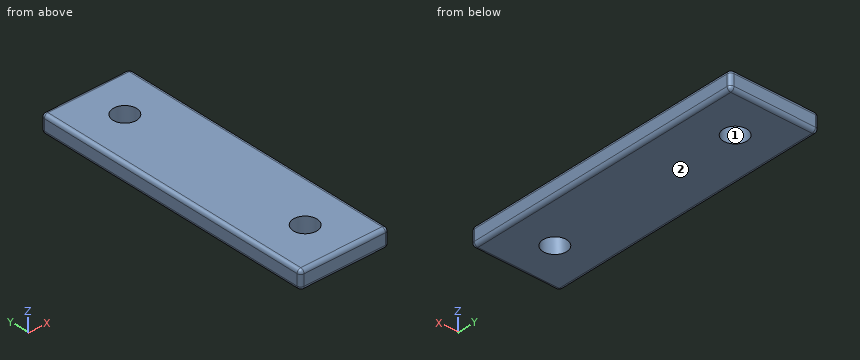
from build123d import *

# Parameters (mm, degrees)
SKETCH1_W           = 48
SKETCH1_H           = 155
BOSS_EXTRUDE1_DEPTH = 10
FILLET1_R           = 2
FILLET2_R           = 2
SKETCH2_R           = 6.4
CUT_EXTRUDE1_DEPTH  = 82.74503043


with BuildPart() as part:
    # Sketch1 → Boss-Extrude1 (new body)
    with BuildSketch(Plane.XY):
        Rectangle(SKETCH1_W, SKETCH1_H)
    extrude(amount=BOSS_EXTRUDE1_DEPTH)

    # Fillet1
    fillet1_edges = [part.edges().sort_by_distance(p)[0] for p in [
        (-24, 0, 10),
        (0, -77.5, 10),
        (24, 0, 10),
        (0, -77.5, 0),
        (-24, 0, 0),
        (0, 77.5, 0),
        (24, 0, 0),
        (0, 77.5, 10),
    ]]
    fillet(fillet1_edges, radius=FILLET1_R)

    # Fillet2
    # the kernel refuses this fillet: 2 mm, written as the material it takes off along each edge
    with BuildSketch(Plane(origin=(-22, 75.5, 8), x_dir=(0, 1, 0), z_dir=(-1, 0, 0))) as fillet2_piece_1_section:
        Polygon((0, 0), (FILLET2_R, 0), (FILLET2_R, -FILLET2_R), (0, -FILLET2_R), align=None)
    fillet2_piece_1 = extrude(amount=FILLET2_R, mode=Mode.PRIVATE)
    fillet2_piece_1 = fillet2_piece_1 - Plane(origin=(-22, 75.5, 8), x_dir=(0, -0.7071067811865475, -0.7071067811865475), z_dir=(-1, 0, 0)) * Sphere(FILLET2_R, mode=Mode.PRIVATE)
    add(fillet2_piece_1, mode=Mode.SUBTRACT)
    with BuildSketch(Plane(origin=(22, 75.5, 8), x_dir=(0, 1, 0), z_dir=(1, 0, 0))) as fillet2_piece_2_section:
        Polygon((0, 0), (FILLET2_R, 0), (FILLET2_R, FILLET2_R), (0, FILLET2_R), align=None)
    fillet2_piece_2 = extrude(amount=FILLET2_R, mode=Mode.PRIVATE)
    fillet2_piece_2 = fillet2_piece_2 - Plane(origin=(22, 75.5, 8), x_dir=(0, -0.7071067811865475, -0.7071067811865475), z_dir=(1, 0, 0)) * Sphere(FILLET2_R, mode=Mode.PRIVATE)
    add(fillet2_piece_2, mode=Mode.SUBTRACT)
    with BuildSketch(Plane(origin=(-22, -75.5, 8), x_dir=(-1, 0, 0), z_dir=(0, -1, 0))) as fillet2_piece_3_section:
        Polygon((0, 0), (FILLET2_R, 0), (FILLET2_R, -FILLET2_R), (0, -FILLET2_R), align=None)
    fillet2_piece_3 = extrude(amount=FILLET2_R, mode=Mode.PRIVATE)
    fillet2_piece_3 = fillet2_piece_3 - Plane(origin=(-22, -75.5, 8), x_dir=(0.7071067811865475, 0, -0.7071067811865475), z_dir=(0, -1, 0)) * Sphere(FILLET2_R, mode=Mode.PRIVATE)
    add(fillet2_piece_3, mode=Mode.SUBTRACT)
    with BuildSketch(Plane(origin=(22, -75.5, 8), x_dir=(1, 0, 0), z_dir=(0, -1, 0))) as fillet2_piece_4_section:
        Polygon((0, 0), (FILLET2_R, 0), (FILLET2_R, FILLET2_R), (0, FILLET2_R), align=None)
    fillet2_piece_4 = extrude(amount=FILLET2_R, mode=Mode.PRIVATE)
    fillet2_piece_4 = fillet2_piece_4 - Plane(origin=(22, -75.5, 8), x_dir=(-0.7071067811865475, 0, -0.7071067811865475), z_dir=(0, -1, 0)) * Sphere(FILLET2_R, mode=Mode.PRIVATE)
    add(fillet2_piece_4, mode=Mode.SUBTRACT)
    with BuildSketch(Plane(origin=(22, -75.5, 2), x_dir=(1, 0, 0), z_dir=(0, -1, 0))) as fillet2_piece_5_section:
        Polygon((0, 0), (FILLET2_R, 0), (FILLET2_R, -FILLET2_R), (0, -FILLET2_R), align=None)
    fillet2_piece_5 = extrude(amount=FILLET2_R, mode=Mode.PRIVATE)
    fillet2_piece_5 = fillet2_piece_5 - Plane(origin=(22, -75.5, 2), x_dir=(-0.7071067811865475, 0, 0.7071067811865475), z_dir=(0, -1, 0)) * Sphere(FILLET2_R, mode=Mode.PRIVATE)
    add(fillet2_piece_5, mode=Mode.SUBTRACT)
    with BuildSketch(Plane(origin=(-22, -75.5, 2), x_dir=(-1, 0, 0), z_dir=(0, -1, 0))) as fillet2_piece_6_section:
        Polygon((0, 0), (FILLET2_R, 0), (FILLET2_R, FILLET2_R), (0, FILLET2_R), align=None)
    fillet2_piece_6 = extrude(amount=FILLET2_R, mode=Mode.PRIVATE)
    fillet2_piece_6 = fillet2_piece_6 - Plane(origin=(-22, -75.5, 2), x_dir=(0.7071067811865475, 0, 0.7071067811865475), z_dir=(0, -1, 0)) * Sphere(FILLET2_R, mode=Mode.PRIVATE)
    add(fillet2_piece_6, mode=Mode.SUBTRACT)
    with BuildSketch(Plane(origin=(22, 75.5, 2), x_dir=(0, 1, 0), z_dir=(1, 0, 0))) as fillet2_piece_7_section:
        Polygon((0, 0), (FILLET2_R, 0), (FILLET2_R, -FILLET2_R), (0, -FILLET2_R), align=None)
    fillet2_piece_7 = extrude(amount=FILLET2_R, mode=Mode.PRIVATE)
    fillet2_piece_7 = fillet2_piece_7 - Plane(origin=(22, 75.5, 2), x_dir=(0, -0.7071067811865475, 0.7071067811865475), z_dir=(1, 0, 0)) * Sphere(FILLET2_R, mode=Mode.PRIVATE)
    add(fillet2_piece_7, mode=Mode.SUBTRACT)
    with BuildSketch(Plane(origin=(-22, 75.5, 2), x_dir=(0, 1, 0), z_dir=(-1, 0, 0))) as fillet2_piece_8_section:
        Polygon((0, 0), (FILLET2_R, 0), (FILLET2_R, FILLET2_R), (0, FILLET2_R), align=None)
    fillet2_piece_8 = extrude(amount=FILLET2_R, mode=Mode.PRIVATE)
    fillet2_piece_8 = fillet2_piece_8 - Plane(origin=(-22, 75.5, 2), x_dir=(0, -0.7071067811865475, 0.7071067811865475), z_dir=(-1, 0, 0)) * Sphere(FILLET2_R, mode=Mode.PRIVATE)
    add(fillet2_piece_8, mode=Mode.SUBTRACT)
    with BuildSketch(Plane(origin=(24, -77.5, 2), x_dir=(-1, 0, 0), z_dir=(0, 0, 1)), Plane(origin=(24, 77.5, 2), x_dir=(0, -1, 0), z_dir=(0, 0, 1))) as fillet2_piece_9:
        with BuildLine():
            CenterArc((FILLET2_R, -FILLET2_R), FILLET2_R, 90, 90)
            Line((0, -FILLET2_R), (0, 0))
            Line((0, 0), (FILLET2_R, 0))
        make_face()
    extrude(amount=6, mode=Mode.SUBTRACT)
    with BuildSketch(Plane(origin=(-24, -77.5, 2), x_dir=(1, 0, 0), z_dir=(0, 0, 1)), Plane(origin=(-24, 77.5, 2), x_dir=(0, -1, 0), z_dir=(0, 0, 1))) as fillet2_piece_10:
        with BuildLine():
            CenterArc((FILLET2_R, FILLET2_R), FILLET2_R, 180, 90)
            Line((0, FILLET2_R), (0, 0))
            Line((0, 0), (FILLET2_R, 0))
        make_face()
    extrude(amount=6, mode=Mode.SUBTRACT)

    # Sketch2 → Cut-Extrude1 (cut, through all)
    with BuildSketch(Plane(origin=(0, 0, 0), x_dir=(-1, 0, 0), z_dir=(0, 0, -1))):
        with Locations((0, 53.85)):
            Circle(SKETCH2_R)
    cut_extrude1 = extrude(amount=-CUT_EXTRUDE1_DEPTH, mode=Mode.SUBTRACT)

    # Mirror2: Cut-Extrude1 across plane
    add(cut_extrude1.mirror(Plane.ZX), mode=Mode.SUBTRACT)


solid = part.part
Geometry: final body of the model. Coordinates: model frame, mm. Face numbers are marked on the shaded views. Give positions to 0.01 mm unless a question says otherwise; leave off trailing zeros. Order: outer loops, then holes, each group sorted by start corner. A loop starts at its lowest first (then second) coordinate and runs counter-clockwise, first axis right, second up. Notation, with made-up numbers: (82, -31) -> (87, -31) arc R24 ccw to (87, -15) -> close; hole circle Ø5 at (78, 27). An arc over 180 degrees is marked (long way). Write each question's results on one line, items separated by ' | '.
1) Cut plane C-C (z = 4). Output: boundary loops of the cut face in (x, y).
Geometry says:
outline: (-24, -75.5) arc R2 ccw to (-22, -77.5) -> (22, -77.5) arc R2 ccw to (24, -75.5) -> (24, 75.5) arc R2 ccw to (22, 77.5) -> (-22, 77.5) arc R2 ccw to (-24, 75.5) -> close; hole circle Ø12.8 at (0, -53.85); hole circle Ø12.8 at (0, 53.85)
2) Cut plane B-B (y = -53.85). Output: boundary loops of the cut face in (x, z), and give its area (3 significant figures).
Geometry says:
outline: (-24, 2) arc R2 ccw to (-22, 0) -> (-6.4, 0) -> (-6.4, 10) -> (-22, 10) arc R2 ccw to (-24, 8) -> close; (6.4, 0) -> (22, 0) arc R2 ccw to (24, 2) -> (24, 8) arc R2 ccw to (22, 10) -> (6.4, 10) -> close | area: 349 mm²
3) Draft query along Y for the marked faces 1 and 2. Return one class per face: released by +Y, released by -Y, zero draft, split by the parting line, or undercut.
Geometry says:
face 1: undercut | face 2: zero draft
4) First-contact query: pin 1 Ø7.5 at (x, y) = (0, -53.85) entering from +Z. Flat tip, straight axial feed; report the tip coordinate or a pass-through.
Geometry says:
pin 1: passes through
5) Line query: line 1 along Y through (x, z) = (0, 6.25); line 2 along X through (y, z) = (-53.85, 5); line 3 along Y through (x, z) = (-2, 1.5). Output: solid intervals per line, ascending.
Geometry says:
line 1: y = -77.5 to -60.25, -47.45 to 47.45, 60.25 to 77.5 | line 2: x = -24 to -6.4, 6.4 to 24 | line 3: y = -77.44 to -59.93, -47.77 to 47.77, 59.93 to 77.44
6) Cut plane A-A (x = 0). Output: boundary loops of the cut face in (y, z).
Geometry says:
outline: (-77.5, 2) arc R2 ccw to (-75.5, 0) -> (-60.25, 0) -> (-60.25, 10) -> (-75.5, 10) arc R2 ccw to (-77.5, 8) -> close; (-47.45, 0) -> (47.45, 0) -> (47.45, 10) -> (-47.45, 10) -> close; (60.25, 0) -> (75.5, 0) arc R2 ccw to (77.5, 2) -> (77.5, 8) arc R2 ccw to (75.5, 10) -> (60.25, 10) -> close
